from build123d import *


with BuildPart() as part:
    # Esboço2 → Revolução1 (revolve)
    with BuildSketch(Plane.XY, mode=Mode.PRIVATE) as revolu_o1_sk:
        with BuildLine():
            Line((0, 0), (0, 29.3))
            Line((0, 29.3), (-0.1, 29.8))
            Line((-0.1, 29.8), (-0.1, 52.16829481))
            ThreePointArc((-0.1, 52.16829481), (-0.097533347, 52.199608972), (-0.090194233, 52.230150722))
            Line((-0.090194233, 52.230150722), (0.427794957, 53.822861152))
            ThreePointArc((0.427794957, 53.822861152), (0.466757595, 53.891883063), (0.529471576, 53.940350248))
            ThreePointArc((0.529471576, 53.940350248), (1.821567106, 54.403034378), (3.185, 54.56))
            Line((3.185, 54.56), (3.185, 0))
            Line((3.185, 0), (0, 0))
        make_face()
    revolve(revolu_o1_sk.sketch.rotate(Axis((3.185, 54.56, 0), (0, -1, 0)), 270), axis=Axis((3.185, 54.56, 0), (0, -1, 0)))


solid = part.part
Verification items for the finished model (mm, model axes). A direction names the side the tool comes from. Coordinates: 2 decimals unless noted, no trailing zeros. Loops run counter-clockwise (first coordinate to the right, second up) from the corner with the lowest first, then second, coordinate; pieces in that order, holes last. Notation, with made-up numbers: (-17.75, 6.25) -> (-1.75, 6.25) arc R23 ccw to (-1.75, 20.25) -> close; hole circle Ø1 at (47, 34). An arc over 180 degrees is marked (long way). Answer as a JSON object with one key per item and string values. Group by question number.
Item 1: Sectioned sample at A-A on z = 0. Record the boundary of the cut face in (x, y) (3 decimals), plus the area to 3 significant figures.
Item 2: Tool access check on faces 1 (the cylindrical face through (0, 15, 0)), 2 (the cylindrical face through (5.18, 41.14, -2.61)). Record the directions out of +Z, -Z, +X, -X, +Y, -Y that give a thin tool (end or side, any length) a straight path to the whole face; none if there is none.
Item 3: Sectioned sample at C-C on y = 22.5. Record the boundary of the cut face in (x, z) (3 decimals).
Item 4: Depth check by flat-ended pin: pin 1 (2 mm diameter, centred on x = 5.5, y = 44, fed in from -Z); pin 2 (1 mm diameter, centred on x = 2, y = 24.5, fed in from -Z). Enter the tip coordinate at first touch or a pass-through.
Item 5: Scan lines: probe 1 along X at (y, z) = (26, -0.25); probe 2 along Z at (x, y) = (1.25, 39); probe 3 along X at (y, z) = (39.5, -0.25). Record each from-to range of solid material in increasing order.
Item 6: Sectioned sample at B-B on y = 43. Record the boundary of the cut face in (x, z) (3 decimals), plus the area to 3 significant figures.
Evaluation:
{
 "1": {"outline": "(-0.1, 29.8) -> (0, 29.3) -> (0, 0) -> (6.37, 0) -> (6.37, 29.3) -> (6.47, 29.8) -> (6.47, 52.168) arc R0.2 ccw to (6.46, 52.23) -> (5.942, 53.823) arc R0.2 ccw to (5.841, 53.94) arc R6 ccw to (0.529, 53.94) arc R0.2 ccw to (0.428, 53.823) -> (-0.09, 52.23) arc R0.2 ccw to (-0.1, 52.168) -> close", "area": "350 mm²"},
 "2": {"face 1": "-Y", "face 2": "+Y, -Y"},
 "3": {"outline": "circle Ø6.37 at (3.185, 0)"},
 "4": {"pin 1": "stops at z = -3.01", "pin 2": "stops at z = -3.11"},
 "5": {"probe 1": "x = 0.01 to 6.36", "probe 2": "z = -2.65 to 2.65", "probe 3": "x = -0.09 to 6.46"},
 "6": {"outline": "circle Ø6.57 at (3.185, 0)", "area": "33.9 mm²"}
}
